Part print with two shaded views. Sizes in mm from the minimum x, y, z corner. A direction names the side the tool comes from. Coordinates: 2 decimals unless noted, no trailing zeros. Order: outer loops, then holes, each group sorted by start corner. A loop starts at its lowest first (then second) coordinate and runs counter-clockwise, first axis right, second up.
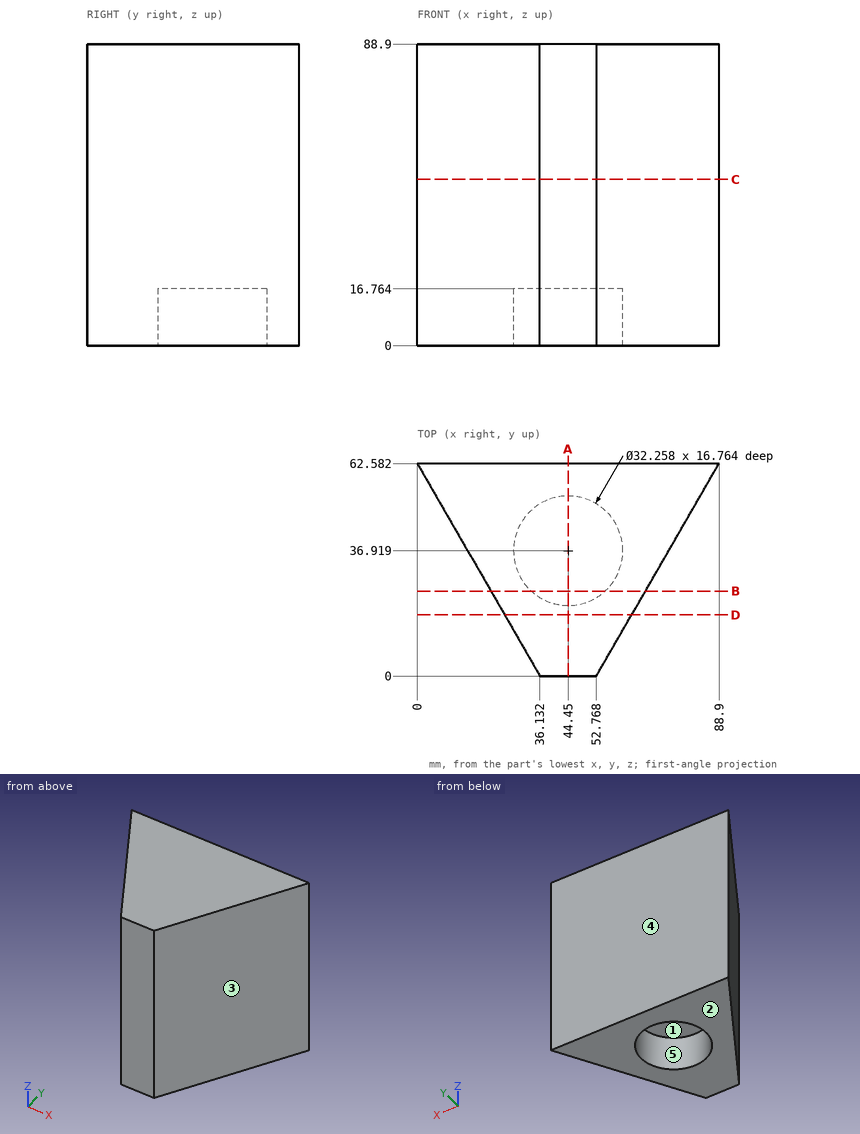
Q1. Cut at D-D on y = 18. Write the cut outline in (x, z).
Results list:
outline: (25.74, 0) - (63.16, 0) - (63.16, 88.9) - (25.74, 88.9) - close
Q2. Wall check: line 1 along Y through (x, z) = (44.45, 5); line 2 along X through (y, z) = (24, 10.5) (1 decimal); line 3 along Z through (x, y) = (41, 22.5). Give the ranges that are in metal, low to high.
Results list:
line 1: y = 0 to 20.79, 53.05 to 62.58
line 2: x = 22.3 to 34.8, 54.1 to 66.6
line 3: z = 16.76 to 88.9
Q3. Cut at B-B on y = 25. Write the cut outline in (x, z).
Results list:
outline: (21.7, 0) - (33.58, 0) - (33.58, 16.76) - (55.32, 16.76) - (55.32, 0) - (67.2, 0) - (67.2, 88.9) - (21.7, 88.9) - close
Q4. Mould opens along Y. For the marked faces 3, 4 and 5 say: pulls with the +Y half, pulls with the -Y half, needs draft (parallel to the pull), parting line crosses it, or undercut.
Results list:
face 3: pulls with the -Y half
face 4: pulls with the +Y half
face 5: undercut
Q5. Which spindle directions (+Z, -Z, +X, -X, +Y, -Y) get a long thin tool onto all of the face, cutting with end or side? Do the marked faces 1 and 2. Say none if no direction does.
Results list:
face 1: -Z
face 2: -Z, +X, -X, +Y, -Y
Q6. Cut at A-A on x = 44.45. Write the cut outline in (y, z), and give its area (3 significant figures).
Results list:
outline: (0, 0) - (20.79, 0) - (20.79, 16.76) - (53.05, 16.76) - (53.05, 0) - (62.58, 0) - (62.58, 88.9) - (0, 88.9) - close
area: 5,020 mm2
Q7. Cut at C-C on z = 49. Write the cut outline in (x, y).
Results list:
outline: (0, 62.58) - (36.13, 0) - (52.77, 0) - (88.9, 62.58) - close
Q8. Pin check, flat tips, straight feed: pin 1 Ø4 at (y, z) = (33, 75.5) entering from -X (1 decimal); pin 2 Ø2 at (y, z) = (25, 36) entering from +X; pin 3 Ø5 at (x, y) = (64, 22.5) entering from -Z; pin 4 Ø2 at (y, z) = (39.5, 16) entering from -X. Stop position of each tip, or through.
Results list:
pin 1: stops at x = 15.9
pin 2: stops at x = 67.78
pin 3: stops at z = 0
pin 4: stops at x = 12.75
